Could you check a few things on this model? Use its own coordinates, in mm. Face numbers are marked on the shaded views. A direction names the side the tool comes from. Round coordinates to 2 decimals unless told otherwise and drop trailing zeros. Loops run counter-clockwise (first coordinate to the right, second up) from the corner with the lowest first, then second, coordinate; pieces in that order, holes last. Notation, with made-up numbers: (22.5, -3) -> (46.5, -3) arc R25 ccw to (46.5, 14) -> close; hole circle Ø8 at (11.25, 84). An arc over 180 degrees is marked (long way). Use CSV: the item, a comma, the result in double quotes. Start each with the question number.
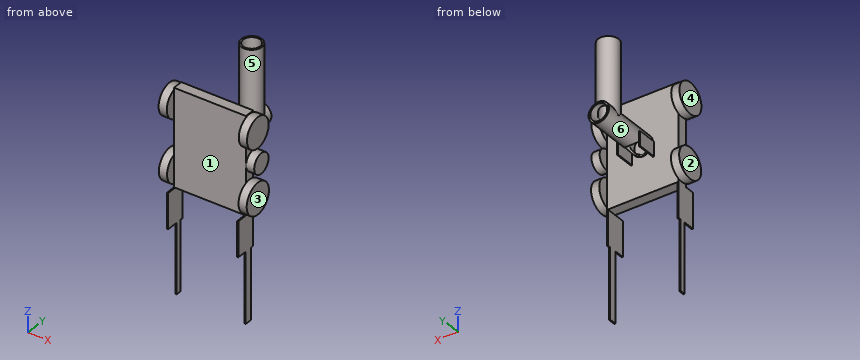
```python
from build123d import *

# Parameters (mm, degrees)
F0_W      = 89.10818398
F0_H      = 120.1675757766
F1_DEPTH  = 12.7
F2_R      = 19.05
F3_DEPTH  = 10.16
F4_R      = 19.05
F5_DEPTH  = 10.16
F6_R      = 18.7667167596
F7_DEPTH  = 10.16
F8_R      = 19.2986234131
F9_DEPTH  = 10.16
F10_R     = 12.4156573735
F11_DEPTH = 10.16
F12_R     = 12.6694142054
F13_DEPTH = 76.2
F14_R     = 12.7449680287
F15_DEPTH = 92.456
F16_R     = 10.4865516495
F17_DEPTH = 76.2
F18_R     = 10.6677127508
F19_DEPTH = 88.9
F20_R     = 11.5560475943
F21_DEPTH = 25.4
F24_W     = 1.3282671571
F24_H     = 25.8222837001
F25_DEPTH = 43.434
F26_W     = 1.4417506754
F26_H     = 24.6515385807
F27_DEPTH = 43.688
F22_W     = 1.255504787
F22_H     = 24.4307331741
F30_DEPTH = 18.034
F23_W     = 1.2999391183
F23_H     = 24.1094622761
F31_DEPTH = 18.034
F36_W     = 1.3282671571
F36_H     = 9.5440435689
F37_DEPTH = 87.376
F38_W     = 1.4417506754
F38_H     = 7.3205276858
F39_DEPTH = 86.36


# Not quite as in the source:
# - the program builds the solid bodies; features that only make, move or delete a surface that nothing else refers to are left out


with BuildPart() as f1:
    # F0 (on Front) → F1 (new body)
    with BuildSketch(Plane.XZ):
        Rectangle(F0_W, F0_H)
    extrude(amount=F1_DEPTH)

    # F2 (on face) → F3 (join)
    with BuildSketch(Plane(origin=(-44.55409199, 0, 0), x_dir=(0, -1, 0), z_dir=(-1, 0, 0))):
        with Locations((6.0873422772, 39.9295948446)):
            Circle(F2_R)
    extrude(amount=F3_DEPTH)

    # F4 (on face) → F5 (join)
    with BuildSketch(Plane(origin=(-44.55409199, 0, 0), x_dir=(0, -1, 0), z_dir=(-1, 0, 0))):
        with Locations((5.5960081518, -38.5527424514)):
            Circle(F4_R)
    extrude(amount=F5_DEPTH)

    # F6 (on face) → F7 (join)
    with BuildSketch(Plane.YZ.offset(44.55409199)):
        with Locations((-6.1870645732, 40.3565391898)):
            Circle(F6_R)
    extrude(amount=F7_DEPTH)

    # F8 (on face) → F9 (join)
    with BuildSketch(Plane.YZ.offset(44.55409199)):
        with Locations((-6.1870645732, -39.2316170037)):
            Circle(F8_R)
    extrude(amount=F9_DEPTH)

    # F10 (on face) → F11 (join)
    with BuildSketch(Plane.YZ.offset(44.55409199)):
        Circle(F10_R)
    extrude(amount=F11_DEPTH)

    # F12 (on face) → F13 (join)
    with BuildSketch(Plane(origin=(0, 0, 0), x_dir=(-1, 0, 0), z_dir=(0, 1, 0))):
        Circle(F12_R)
    extrude(amount=F13_DEPTH)

    # F14 (on Top) → F15 (join)
    with BuildSketch(Plane.XY):
        with Locations((0, 59.6004612744)):
            Circle(F14_R)
    extrude(amount=F15_DEPTH)

    # F16 (on face) → F17 (cut)
    with BuildSketch(Plane(origin=(0, 76.2, 0), x_dir=(-1, 0, 0), z_dir=(0, 1, 0))):
        Circle(F16_R)
    extrude(amount=-F17_DEPTH, mode=Mode.SUBTRACT)

    # F18 (on face) → F19 (cut)
    with BuildSketch(Plane.XY.offset(92.456)):
        with Locations((0, 59.6004612744)):
            Circle(F18_R)
    extrude(amount=-F19_DEPTH, mode=Mode.SUBTRACT)

    # F20 (on Top) → F21 (cut)
    with BuildSketch(Plane.XY):
        with Locations((0, 12.4179841951)):
            Circle(F20_R)
    extrude(amount=-F21_DEPTH, mode=Mode.SUBTRACT)

    # F24 (on face) → F25 (join)
    with BuildSketch(Plane(origin=(0, 0, -60.0837878883), x_dir=(1, 0, 0), z_dir=(0, 0, -1))):
        with Locations((43.8899584115, 12.9111418501)):
            Rectangle(F24_W, F24_H)
    extrude(amount=F25_DEPTH)

    # F26 (on face) → F27 (join)
    with BuildSketch(Plane(origin=(0, 0, -60.0837878883), x_dir=(1, 0, 0), z_dir=(0, 0, -1))):
        with Locations((-43.8332166523, 12.3257692903)):
            Rectangle(F26_W, F26_H)
    extrude(amount=F27_DEPTH)

    # F22 (on Top) → F30 (join)
    with BuildSketch(Plane.XY):
        with Locations((14.0256239101, 12.215366587)):
            Rectangle(F22_W, F22_H)
    extrude(amount=-F30_DEPTH)

    # F23 (on Top) → F31 (join)
    with BuildSketch(Plane.XY):
        with Locations((-13.2890497334, 12.0547311381)):
            Rectangle(F23_W, F23_H)
    extrude(amount=-F31_DEPTH)

    # F36 (on face) → F37 (join)
    with BuildSketch(Plane(origin=(0, 0, -103.5177878883), x_dir=(1, 0, 0), z_dir=(0, 0, -1))):
        with Locations((43.8899584115, 8.1391200656)):
            Rectangle(F36_W, F36_H)
    extrude(amount=F37_DEPTH)

    # F38 (on face) → F39 (join)
    with BuildSketch(Plane(origin=(0, 0, -103.7717878883), x_dir=(1, 0, 0), z_dir=(0, 0, -1))):
        with Locations((-43.8332166523, 6.7722700769)):
            Rectangle(F38_W, F38_H)
    extrude(amount=F39_DEPTH)


solid = f1.part
```
1. Suppose I cut it at B-B (z = -124.5). List the corners of the cut face in (x, y) for me, then the cut area to 3 significant figures.
2. Suppose I cut it at C-C (y = 20). List the corners of the cut face in (x, z) for me, then the cut area to 3 significant figures.
3. Will these pins go through, and if not, where does the flat tip stop? pin 1 (0.9 mm diameter, centred on x = -11, y = 11.5, fed in from -Z); pin 2 (17 mm diameter, centred on x = 0, z = 0, fed in from -Y); pin 3 (4 mm diameter, centred on y = 55.5, z = 29, fed in from +X); pin 4 (3 mm diameter, centred on x = 15, y = 61, fed in from -Z).
4. If I drill on L1, parallel to Y at x = 0, z = 37; L2, parallel to X at y = 52, z = 0; L3, parallel to X at y = 3, z = -39, over which ranges is the centre line in solid material (lowest first)?
5. We'd pull the mould along X, two halves only. Please class the marked faces 1, 2 and 3: pulls with the +X half, pulls with the -X half, needs draft (parallel to the pull), parting line crosses it, or undercut.
6. Suppose I cut it at D-D (z = -27). List the corners of the cut face in (x, y) for me.
7. For the marked faces 4, 5 and 6, which set-ups out of +Z, -Z, +X, -X, +Y, -Y let a thin tool reach every point of the face, with its end or its side?
8. Suppose I cut it at A-A (x = 0). List the corners of the cut face in (y, z) for me.
Geometry check:
1,outline,"(-44.55, -10.43) -> (-43.11, -10.43) -> (-43.11, -3.11) -> (-44.55, -3.11) -> close; (43.23, -12.91) -> (44.55, -12.91) -> (44.55, -3.37) -> (43.23, -3.37) -> close"
1,area,"23.2 mm²"
2,outline,"(-13.94, -18.03) -> (-12.64, -18.03) -> (-12.64, -0.88) arc R12.67 ccw to (-8.72, -9.19) -> (-8.72, -5.82) arc R10.49 cw (long way) to (8.72, -5.82) -> (8.72, -9.19) arc R12.67 ccw (long way) to (-12.67, 0) -> (-13.94, 0) -> close; (13.4, -18.03) -> (14.65, -18.03) -> (14.65, 0) -> (13.4, 0) -> close"
2,area,"162 mm²"
3,pin 1,"stops at z = 0"
3,pin 2,"stops at y = -12.7"
3,pin 3,"stops at x = 12.57"
3,pin 4,"passes through"
4,L1,"y = -12.7 to 0, 46.86 to 48.93, 70.27 to 72.35"
4,L2,"x = -12.67 to -10.49, 10.49 to 12.67"
4,L3,"x = -54.71 to -44.55, 44.55 to 54.71"
5,face 1,"undercut"
5,face 2,"pulls with the -X half"
5,face 3,"pulls with the +X half"
6,outline,"(-54.71, -20.74) -> (-44.55, -20.74) -> (-44.55, -12.7) -> (44.55, -12.7) -> (44.55, -21.11) -> (54.71, -21.11) -> (54.71, 8.74) -> (44.55, 8.74) -> (44.55, 0) -> (-44.55, 0) -> (-44.55, 9.55) -> (-54.71, 9.55) -> close"
7,face 4,"+Z, -Z, -X, +Y, -Y"
7,face 5,"+Z"
7,face 6,"none"
8,outline,"(-12.7, -60.08) -> (0, -60.08) -> (0, -12.67) -> (0.86, -12.67) -> (0.86, -10.49) -> (0, -10.49) -> (0, 10.49) -> (48.93, 10.49) -> (48.93, 92.46) -> (46.86, 92.46) -> (46.86, 12.67) -> (0, 12.67) -> (0, 60.08) -> (-12.7, 60.08) -> close; (23.97, -12.67) -> (76.2, -12.67) -> (76.2, -10.49) -> (23.97, -10.49) -> close; (70.27, 10.49) -> (76.2, 10.49) -> (76.2, 12.67) -> (72.35, 12.67) -> (72.35, 92.46) -> (70.27, 92.46) -> close"
